Read the model definition and answer for the solid it produces. Units are mm, in the model's axes. A direction names the side the tool comes from. Give positions to 0.01 mm unless a question says otherwise; leave off trailing zeros. Write each loop counter-clockwise with the first axis right and the second up, starting at its lowest first coordinate (ties: lowest second). Pieces come first, ordered by that corner, then holes.
```python
from build123d import *

# Parameters (mm, degrees)
BOSS_EXTRUDE1_DEPTH     = 27.5
CUT_EXTRUDE1_DEPTH      = 91.251038775
CUT_EXTRUDE1_DEPTH_BACK = 91.251038775
SKETCH3_W               = 37
SKETCH3_H               = 20
CUT_EXTRUDE2_REACH      = 92.251


with BuildPart() as part:
    # Sketch1 → Boss-Extrude1 (new, symmetric)
    with BuildSketch(Plane.XY):
        with BuildLine():
            Line((-62.5, 0), (62.5, 0))
            Line((62.5, 0), (62.5, 10))
            Line((62.5, 10), (75, 10))
            ThreePointArc((75, 10), (65.627416998, 32.627416998), (43, 42))
            Line((43, 42), (-43, 42))
            ThreePointArc((-43, 42), (-65.627416998, 32.627416998), (-75, 10))
            Line((-75, 10), (-62.5, 10))
            Line((-62.5, 10), (-62.5, 0))
        make_face()
    extrude(amount=BOSS_EXTRUDE1_DEPTH, both=True)

    # Sketch3 → Cut-Extrude1 (cut, two sides: drawn at the far end of the back side and taken through both)
    with BuildSketch(Plane(origin=(0, 0, 0), x_dir=(0, 0, -1), z_dir=(1, 0, 0)).offset(-CUT_EXTRUDE1_DEPTH_BACK)):
        with Locations((0, 32)):
            Rectangle(SKETCH3_W, SKETCH3_H)
    extrude(amount=CUT_EXTRUDE1_DEPTH + CUT_EXTRUDE1_DEPTH_BACK, mode=Mode.SUBTRACT)

    # Sketch2 → Cut-Extrude2 (cut, up to next)
    with BuildSketch(Plane(origin=(0, 42, 0), x_dir=(1, 0, 0), z_dir=(0, 1, 0)), mode=Mode.PRIVATE) as cut_extrude2_sk1:
        with BuildLine():
            Line((-14, 6), (-47, 6))
            ThreePointArc((-47, 6), (-53, 0), (-47, -6))
            Line((-47, -6), (-14, -6))
            ThreePointArc((-14, -6), (-8, 0), (-14, 6))
        make_face()
    cut_extrude2_tool1 = extrude(cut_extrude2_sk1.sketch, amount=-CUT_EXTRUDE2_REACH, mode=Mode.PRIVATE) & part.part
    # Sketch2 → Cut-Extrude2 (cut, up to next)
    with BuildSketch(Plane(origin=(0, 42, 0), x_dir=(1, 0, 0), z_dir=(0, 1, 0)), mode=Mode.PRIVATE) as cut_extrude2_sk2:
        with BuildLine():
            Line((14, 6), (47, 6))
            ThreePointArc((47, 6), (53, 0), (47, -6))
            Line((47, -6), (14, -6))
            ThreePointArc((14, -6), (8, 0), (14, 6))
        make_face()
    cut_extrude2_tool2 = extrude(cut_extrude2_sk2.sketch, amount=-CUT_EXTRUDE2_REACH, mode=Mode.PRIVATE) & part.part
    add(cut_extrude2_tool1.solids().sort_by_distance((-30.5, 42, 0))[0], mode=Mode.SUBTRACT)
    add(cut_extrude2_tool2.solids().sort_by_distance((30.5, 42, 0))[0], mode=Mode.SUBTRACT)


solid = part.part
```
Item 1: Section B-B (z = 21) is taken. Write down the section's boundary in (x, y).
Result set:
outline: (-75, 10) - (-62.5, 10) - (-62.5, 0) - (62.5, 0) - (62.5, 10) - (75, 10) arc R32 ccw to (43, 42) - (-43, 42) arc R32 ccw to start
Item 2: Which of the six approach directions +Z, -Z, +X, -X, +Y, -Y give full straight-line access (tool end or side, diameter ignored) to faces 1 (the flat face through (-30, 11, -6)), 2 (the flat face through (62.5, 5, 0)), 3 (the flat face through (-1, 22, 0)), 4 (the flat face through (-69, 10, 0))?
Result set:
face 1: +Y, -Y
face 2: +Z, -Z, +X, -Y
face 3: +X, -X, +Y
face 4: +Z, -Z, -X, -Y
Item 3: Section D-D (x = -49) is taken. Write down the section's boundary in (y, z).
Result set:
outline: (0, -27.5) - (41.43, -27.5) - (41.43, -18.5) - (22, -18.5) - (22, -5.66) - (0, -5.66) - close; (0, 5.66) - (22, 5.66) - (22, 18.5) - (41.43, 18.5) - (41.43, 27.5) - (0, 27.5) - close
Item 4: Section A-A (y = 3.5) is taken. Write down the section's boundary in (x, z).
Result set:
outline: (-62.5, -27.5) - (62.5, -27.5) - (62.5, 27.5) - (-62.5, 27.5) - close; hole (-47, -6) - (-14, -6) arc R6 ccw to (-14, 6) - (-47, 6) arc R6 ccw to start; hole (14, -6) - (47, -6) arc R6 ccw to (47, 6) - (14, 6) arc R6 ccw to start
Item 5: Each of these flat-tipped pins is pushed along its axis until it touches: pin 1 Ø8 at (x, z) = (-50.5, 0) entering from +Y; pin 2 Ø10 at (x, z) = (66.5, 9.5) entering from -Y; pin 3 Ø8 at (y, z) = (25.5, 17) entering from -X; pin 4 Ø1 at (y, z) = (12.5, -0.5) entering from +X. Where does it stop, or does it pass through?
Result set:
pin 1: stops at y = 22
pin 2: stops at y = 0
pin 3: stops at x = -72.86
pin 4: stops at x = 74.94
Item 6: Find the intervals of material crossed by line 1 along Z through (x, y) = (-6.5, 29); line 2 along Z through (x, y) = (-13.5, 5.5); line 3 along X through (y, z) = (6, 5), in increasing order.
Result set:
line 1: z = -27.5 to -18.5, 18.5 to 27.5
line 2: z = -27.5 to -5.98, 5.98 to 27.5
line 3: x = -62.5 to -50.32, -10.68 to 10.68, 50.32 to 62.5
Item 7: Determine the mould class of faces 5 (the flat face through (69, 10, 0)), 6 (the cylindrical face through (-53, 11, 0)) for opening direction Z: pulls with the +Z half, pulls with the -Z half, needs draft (parallel to the pull), parting line crosses it, or undercut.
Result set:
face 5: needs draft
face 6: undercut
Item 8: Section C-C (y = 36) is taken. Write down the section's boundary in (x, z).
Result set:
outline: (-61.65, -27.5) - (61.65, -27.5) - (61.65, -18.5) - (-61.65, -18.5) - close; (-61.65, 18.5) - (61.65, 18.5) - (61.65, 27.5) - (-61.65, 27.5) - close
